Answer from the drawing. Dimensions are ordinates in mm from the lowest x, y and z of the part. A direction names the side the tool comes from. Coordinates: 2 decimals unless noted, no trailing zeros. Order: outer loops, then holes, each group sorted by start corner. A loop starts at its lowest first (then second) coordinate and runs counter-clockwise, first axis right, second up. Notation, with made-up numbers: (-35.5, 31) - (-19.5, 31) arc R4 cw to (-19.5, 35) - close; hole circle Ø3 at (-7, -18). An arc over 180 degrees is marked (long way). Use a Markdown table: item, result. Add a question column.
Item 1: Find the intervals of material crossed by line 1 along Y through (x, z) = (4.75, 5.5); line 2 along Y through (x, z) = (9, 3.6); line 3 along X through (y, z) = (12.5, 5.5), in increasing order.
Item 2: The part is cut by section D-D, the plane z = 1.5. Give the vertices of the cut face in (x, y).
Item 3: The part is cut by section C-C, the plane z = 3.75. Give the vertices of the cut face in (x, y).
Item 4: For the marked faces 1 and 2, determine the directions among +Z, -Z, +X, -X, +Y, -Y from which every point of the face is accessible in a straight line to the end or side of a thin tool.
Item 5: The part is cut by section A-A, the plane y = 9. Give the vertices of the cut face in (x, z), then the cut area to 3 significant figures.
Item 6: Flat-ended cylindrical pins translate along their axes: P1, Ø2, axis at x = 11.5, z = 1.5, coming from the +Y side; P2, Ø1, axis at y = 11, z = 2.5, coming from the -X side; P3, Ø4, axis at y = 14, z = 2, coming from the +X side; P4, Ø8, axis at x = 13, y = 6, coming from the -Z side. Find the tip coordinate at first contact, or state that the pin passes through.
Item 7: The mould has two halves that part along X. Classify the marked faces 3, 4 and 5: released by +X, released by -X, zero draft, split by the parting line, or undercut.
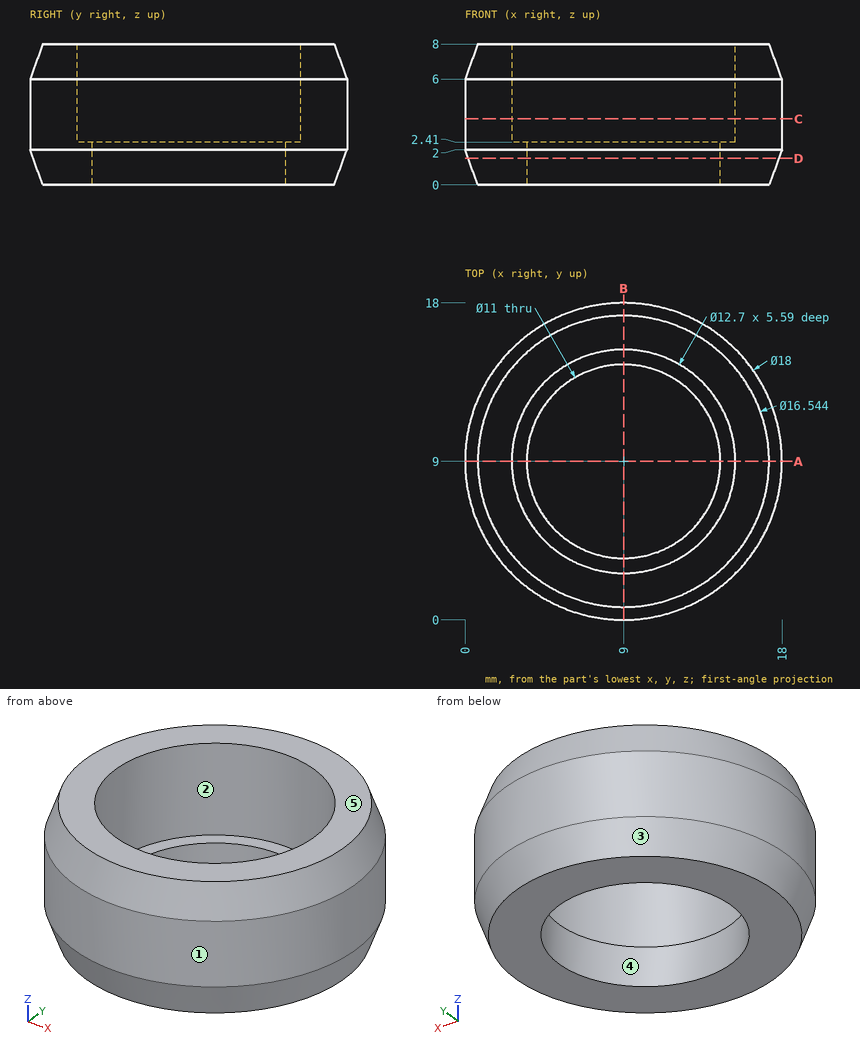
Solution:
| question | item | result |
|---|---|---|
| 1 | line 1 | y = 1.07 to 4.28, 13.72 to 16.93 |
| 1 | line 2 | y = 0 to 2.65, 15.35 to 18 |
| 1 | line 3 | x = 0.71 to 3.7, 14.3 to 17.29 |
| 2 | outline | circle Ø17.64 at (9, 9); hole circle Ø11 at (9, 9) |
| 3 | outline | circle Ø18 at (9, 9); hole circle Ø12.7 at (9, 9) |
| 4 | face 1 | +Z, -Z |
| 4 | face 2 | +Z |
| 5 | outline | (0, 2) - (0.73, 0) - (3.5, 0) - (3.5, 2.41) - (2.65, 2.41) - (2.65, 8) - (0.73, 8) - (0, 6) - close; (14.5, 0) - (17.27, 0) - (18, 2) - (18, 6) - (17.27, 8) - (15.35, 8) - (15.35, 2.41) - (14.5, 2.41) - close |
| 5 | area | 43.6 mm2 |
| 6 | P1 | stops at y = 17.85 |
| 6 | P2 | stops at x = 0.13 |
| 6 | P3 | stops at x = 17.49 |
| 6 | P4 | stops at z = 0 |
| 7 | face 3 | split by the parting line |
| 7 | face 4 | undercut |
| 7 | face 5 | zero draft |
